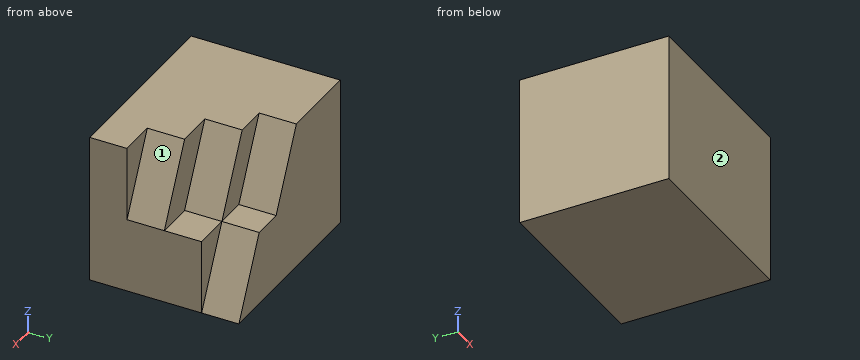
```python
from build123d import *

# Parameters (mm, degrees)
SKETCH1_W           = 50
SKETCH1_H           = 40
BOSS_EXTRUDE1_DEPTH = 40
CUT_EXTRUDE1_DEPTH  = 30
CUT_EXTRUDE2_DEPTH  = 20
CUT_EXTRUDE3_DEPTH  = 10
CUT_EXTRUDE4_DEPTH  = 10


with BuildPart() as part:
    # Sketch1 → Boss-Extrude1 (new body)
    with BuildSketch(Plane(origin=(0, 0, 0), x_dir=(1, 0, 0), z_dir=(0, 1, 0))):
        Rectangle(SKETCH1_W, SKETCH1_H)
    extrude(amount=BOSS_EXTRUDE1_DEPTH)

    # Sketch2 → Cut-Extrude1 (cut)
    with BuildSketch(Plane(origin=(0, 40, 0), x_dir=(1, 0, 0), z_dir=(0, 1, 0))):
        Polygon((25, 0), (15, -20), (25, -20), align=None)
    extrude(amount=-CUT_EXTRUDE1_DEPTH, mode=Mode.SUBTRACT)

    # Sketch3 → Cut-Extrude2 (cut)
    with BuildSketch(Plane(origin=(0, 40, 0), x_dir=(1, 0, 0), z_dir=(0, 1, 0))):
        Polygon((15, 0), (5, -20), (15, -20), (25, 0), align=None)
    extrude(amount=-CUT_EXTRUDE2_DEPTH, mode=Mode.SUBTRACT)

    # Sketch4 → Cut-Extrude3 (cut)
    with BuildSketch(Plane(origin=(0, 40, 0), x_dir=(1, 0, 0), z_dir=(0, 1, 0))):
        Polygon((25, 20), (15, 0), (25, 0), align=None)
    extrude(amount=-CUT_EXTRUDE3_DEPTH, mode=Mode.SUBTRACT)

    # Sketch5 → Cut-Extrude4 (cut)
    with BuildSketch(Plane(origin=(0, 40, 0), x_dir=(1, 0, 0), z_dir=(0, 1, 0))):
        Polygon((15, 0), (6.643581927, 0), (-3.356418073, -20), (5, -20), align=None)
    extrude(amount=-CUT_EXTRUDE4_DEPTH, mode=Mode.SUBTRACT)


solid = part.part
```
Geometry: final body of the model. Coordinates: model frame, mm. Face numbers are marked on the shaded views. A direction names the side the tool comes from. Round coordinates to 2 decimals unless told otherwise and drop trailing zeros. Write each loop counter-clockwise with the first axis right and the second up, starting at its lowest first coordinate (ties: lowest second). Pieces come first, ordered by that corner, then holes.
Item 1: Section query C-C (z = -6). Return loops of the section in (x, y).
Item 2: Set-up query: the marked faces 1 and 2. Return all of +Z, -Z, +X, -X, +Y, -Y with unobstructed straight access to the full face (end or side cutting, diameter ignored); none if empty.
Item 3: Section query A-A (x = 10). Return loops of the section in (y, z), plus the area to 3 significant figures.
Item 4: Section query D-D (x = 21). Return loops of the section in (y, z), plus the area to 3 significant figures.
Item 5: Section query B-B (y = 28.5). Return loops of the section in (x, z).
Item 6: Material intervals for L1, parallel to Y at x = 20, z = 5; L2, parallel to Y at x = 3.5, z = 7; L3, parallel to Z at x = 23.5, y = 21.5, sorted ascending.
Item 7: Pin query (flat end, axial travel): P1, Ø9, axis at x = 4, z = 8, coming from the +Y side; P2, Ø3, axis at x = 21, z = 11, coming from the +Y side; P3, Ø2.5, axis at x = 10, y = 36.5, coming from the +Z side. Return the tip coordinate at first contact, or that it passes through.
Completed:
1. outline: (-25, 0) - (25, 0) - (25, 30) - (18, 30) - (18, 40) - (-25, 40) - close
2. face 1: +Z, +X, +Y
2. face 2: +Z, -Z, +X, -X, -Y
3. outline: (0, -20) - (40, -20) - (40, 0) - (30, 0) - (30, 10) - (20, 10) - (20, 20) - (0, 20) - close
3. area: 1,300 mm2
4. outline: (0, -20) - (40, -20) - (40, -12) - (30, -12) - (30, 0) - (20, 0) - (20, 8) - (10, 8) - (10, 20) - (0, 20) - close
4. area: 960 mm2
5. outline: (-25, -20) - (25, -20) - (25, 0) - (15, 0) - (5, 20) - (-25, 20) - close
6. L1: y = 0 to 20
6. L2: y = 0 to 30
6. L3: z = -20 to 0
7. P1: stops at y = 40
7. P2: stops at y = 20
7. P3: stops at z = 0
